from build123d import *

# Parameters (mm, degrees)
SKETCH_1_W              = 260
SKETCH_1_H              = 206
EXTRUDE_1_DEPTH         = 3
HOLE_WIZARD_3_2_3_2_1_D = 3.2
HOLE_WIZARD_3_2_3_2_2_D = 3.2
HOLE_WIZARD_3_2_3_2_4_D = 3.2
HOLE_WIZARD_4_2_4_2_1_D = 4.2
MIRROR_2_COPY_1_D       = 4.2
CUT_EXTRUDE_1_DEPTH     = 244.608292141
FILLET_1_R              = 2


with BuildPart() as part:
    # 草图1 → 凸台-拉伸1 (new body)
    with BuildSketch(Plane(origin=(0, 0, 0), x_dir=(1, 0, 0), z_dir=(0, 1, 0))):
        with Locations((0, 103)):
            Rectangle(SKETCH_1_W, SKETCH_1_H)
    extrude(amount=EXTRUDE_1_DEPTH)

    # Ø3.2 (3.2) 直径孔1 (through all)
    with Locations(Plane(origin=(-15, 0, -136), x_dir=(0, 0, -1), z_dir=(0, -1, 0))):
        with Locations((0, 0), (-22, 0), (0, -75), (-22, -75)):
            Hole(HOLE_WIZARD_3_2_3_2_1_D / 2)

    # Ø3.2 (3.2) 直径孔2 (through all)
    with Locations(Plane(origin=(45, 0, -26), x_dir=(0, 0, -1), z_dir=(0, -1, 0))):
        with Locations((0, 0), (0, 40), (140, 0), (140, 40)):
            Hole(HOLE_WIZARD_3_2_3_2_2_D / 2)

    # Ø3.2 (3.2) 直径孔4 (through all)
    with Locations(Plane(origin=(-125, 0, -23), x_dir=(0, 0, -1), z_dir=(0, -1, 0))):
        with Locations((0, 0), (20, 0), (140, 0), (160, 0), (140, 250), (160, 250), (20, 250), (0, 250)):
            Hole(HOLE_WIZARD_3_2_3_2_4_D / 2)

    # Ø4.2 (4.2) 直径孔1 (through all)
    with Locations(Plane(origin=(-60, 0, -201), x_dir=(0, 0, -1), z_dir=(0, -1, 0))):
        with Locations((0, 0), (0, -25)):
            hole_wizard_4_2_4_2_1 = Hole(HOLE_WIZARD_4_2_4_2_1_D / 2)

    # 镜向1: Ø4.2 (4.2) 直径孔1 across plane
    add(hole_wizard_4_2_4_2_1.mirror(Plane(origin=(0, 0, 0), x_dir=(0, 0, 1), z_dir=(1, 0, 0))), mode=Mode.SUBTRACT)

    # 镜向2: Ø4.2 (4.2) 直径孔1 across plane
    add(hole_wizard_4_2_4_2_1.mirror(Plane.XY.offset(-103)), mode=Mode.SUBTRACT)

    # 镜向2 copy 1 (through all)
    with Locations(Plane(origin=(60, 0, -5), x_dir=(0, 0, 1), z_dir=(0, -1, 0))):
        with Locations((0, 0), (0, -25)):
            Hole(MIRROR_2_COPY_1_D / 2)

    # 草图11 → 切除-拉伸1 (cut, through all)
    with BuildSketch(Plane.XZ):
        Polygon((-110, -20), (-110, -90), (-64.432146014, -20), align=None)
        Polygon((-52.5, -20), (-98.067853986, -90), (-8.067853986, -90), align=None)
        Polygon((-40.655587213, -20), (3.776558802, -90), (3.776558802, -20), align=None)
        Polygon((18.776558802, -145), (115, -145), (115, -44.462623892), align=None)
        Polygon((-110, -145), (-13.228905706, -145), (-110, -174.76877079), align=None)
        Polygon((-112.49908843, -186), (3.776558802, -186), (3.776558802, -150.23122921), align=None)
        Polygon((18.776558802, -30), (18.776558802, -130.537376108), (115, -30), align=None)
    extrude(amount=-CUT_EXTRUDE_1_DEPTH, mode=Mode.SUBTRACT)

    # 圆角1
    fillet_1_edges = [part.edges().sort_by_distance(p)[0] for p in [
        (115, 1.5, -30),
        (18.776558802, 1.5, -130.537376108),
        (18.776558802, 1.5, -30),
        (18.776558802, 1.5, -145),
        (115, 1.5, -44.462623892),
        (115, 1.5, -145),
        (-110, 1.5, -174.76877079),
        (-110, 1.5, -145),
        (-13.228905706, 1.5, -145),
        (3.776558802, 1.5, -150.23122921),
        (3.776558802, 1.5, -186),
        (-112.49908843, 1.5, -186),
        (-52.5, 1.5, -20),
        (-8.067853986, 1.5, -90),
        (-98.067853986, 1.5, -90),
        (-40.655587213, 1.5, -20),
        (3.776558802, 1.5, -20),
        (3.776558802, 1.5, -90),
        (-110, 1.5, -20),
        (-64.432146014, 1.5, -20),
        (-110, 1.5, -90),
    ]]
    fillet(fillet_1_edges, radius=FILLET_1_R)


solid = part.part
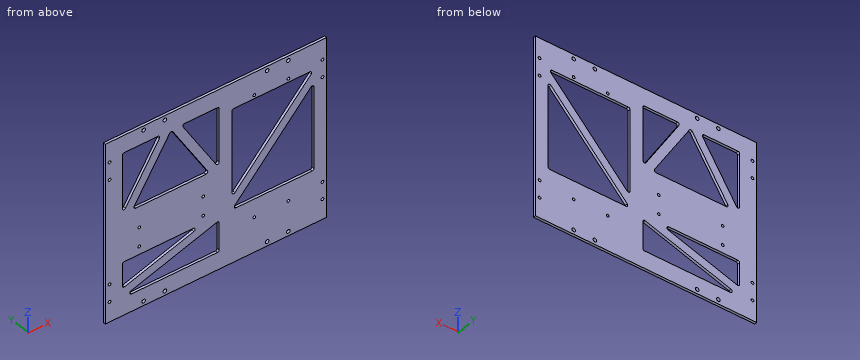
Could you check a few things on this model? Use its own coordinates, in mm. Coordinates: 2 decimals unless noted, no trailing zeros. Loops run counter-clockwise (first coordinate to the right, second up) from the corner with the lowest first, then second, coordinate; pieces in that order, holes last.
1. For P1, Ø4, axis at x = 125, z = -23, coming from the -Y side; P2, Ø2.5, axis at x = 60, z = -201, coming from the -Y side, each with a flat end and sliding along its axis, tell me the tip position at first contact or that it passes through.
2. Imagine slicing it at A-A (z = -79). Please give me the cut outline in (x, y), and give its area (3 significant figures).
3. Imagine slicing it at C-C (x = 31). Please give me the cut outline in (y, z), and give its area (3 significant figures).
4. Imagine slicing it at B-B (z = -177.5). Please give me the cut outline in (x, y), and give its area (3 significant figures).
5. I need wall thicknesses on L1, parallel to Z at x = 24, y = 2.1; L2, parallel to Z at x = 92, y = 2.85; L3, parallel to Z at x = -70, y = 2.85. Which ranges of each line are inside material? Lowest first, please.
6. Imagine slicing it at D-D (y = 1.75). Give the number of separate pieces and of enclosed holes in the cut face, and give its area (3 significant figures).
Computed values:
1. P1: stops at y = 0
1. P2: passes through
2. outline: (-130, 0) - (-110, 0) - (-110, 3) - (-130, 3) - close; (-102.84, 0) - (-90.91, 0) - (-90.91, 3) - (-102.84, 3) - close; (-15.05, 0) - (-3.21, 0) - (-3.21, 3) - (-15.05, 3) - close; (3.78, 0) - (18.78, 0) - (18.78, 3) - (3.78, 3) - close; (68.1, 0) - (81.94, 0) - (81.94, 3) - (68.1, 3) - close; (115, 0) - (130, 0) - (130, 3) - (115, 3) - close
2. area: 263 mm2
3. outline: (0, -206) - (3, -206) - (3, -145) - (0, -145) - close; (0, -132.23) - (3, -132.23) - (3, -117.77) - (0, -117.77) - close; (0, -30) - (3, -30) - (3, 0) - (0, 0) - close
3. area: 316 mm2
4. outline: (-130, 0) - (-84.87, 0) - (-84.87, 3) - (-130, 3) - close; (3.78, 0) - (130, 0) - (130, 3) - (3.78, 3) - close
4. area: 514 mm2
5. L1: z = -206 to -145, -139.54 to -125.08, -30 to 0
5. L2: z = -206 to -145, -68.49 to -54.03, -30 to 0
5. L3: z = -206 to -186, -172.93 to -162.46, -145 to -90, -46.88 to -28.55, -20 to 0
6. separate pieces: 1
6. enclosed holes: 31
6. area: 33,900 mm2
